Design review of the part built by this model. Coordinates are the model's own, in mm. Give positions to 0.01 mm unless a question says otherwise; leave off trailing zeros. Order: outer loops, then holes, each group sorted by start corner. A loop starts at its lowest first (then second) coordinate and runs counter-clockwise, first axis right, second up. Notation, with made-up numbers: (52, -3) -> (103, -3) arc R32 cw to (103, 28) -> close; hole circle Ø11 at (-31, 53.5). An arc over 180 degrees is marked (long way). Return JSON: item names as keys, results as strings.
```python
from build123d import *

# Parameters (mm, degrees)
SKETCH_1_W          = 31
SKETCH_1_H          = 6
EXTRUDE_1_DEPTH     = 2.5
SKETCH_2_R          = 1.1
CUT_EXTRUDE_1_DEPTH = 32.608171111
SKETCH_3_R          = 0.6
CUT_EXTRUDE_2_DEPTH = 32.608171111
FILLET_1_R          = 2


with BuildPart() as part:
    # 草图1 → 凸台-拉伸1 (new body)
    with BuildSketch(Plane(origin=(0, 0, 0), x_dir=(1, 0, 0), z_dir=(0, 1, 0))):
        with Locations((15.5, -2.64149634)):
            Rectangle(SKETCH_1_W, SKETCH_1_H)
    extrude(amount=EXTRUDE_1_DEPTH)

    # 草图2 → 切除-拉伸1 (cut, through all)
    with BuildSketch(Plane(origin=(0, 2.5, 0), x_dir=(1, 0, 0), z_dir=(0, 1, 0))):
        with Locations(Location((3, -2.64149634, 0), (0, 0, 270))):
            Circle(SKETCH_2_R)
        with Locations(Location((17, -2.64149634, 0), (0, 0, 270))):
            Circle(SKETCH_2_R)
    extrude(amount=-CUT_EXTRUDE_1_DEPTH, mode=Mode.SUBTRACT)

    # 草图3 → 切除-拉伸2 (cut, through all)
    with BuildSketch(Plane(origin=(0, 2.5, 0), x_dir=(1, 0, 0), z_dir=(0, 1, 0))):
        with Locations(Location((28.5, -2.64149634, 0), (0, 0, 270))):
            Circle(SKETCH_3_R)
    extrude(amount=-CUT_EXTRUDE_2_DEPTH, mode=Mode.SUBTRACT)

    # 圆角1
    fillet_1_edges = [part.edges().sort_by_distance(p)[0] for p in [
        (0, 1.25, -0.35850366),
        (31, 1.25, -0.35850366),
        (31, 1.25, 5.64149634),
        (0, 1.25, 5.64149634),
    ]]
    fillet(fillet_1_edges, radius=FILLET_1_R)


solid = part.part
```
Item 1: For pin 1 (1 mm diameter, centred on x = 28.5, z = 2.64, fed in from +Y), flat-tipped, find the tip position at first contact; note if it passes through.
Result set:
{"pin 1": "passes through"}
Item 2: Add section C-C (y = 0.35). Give the boundary of the cut face in (x, z).
Result set:
{"outline": "(0, 1.64) arc R2 ccw to (2, -0.36) -> (29, -0.36) arc R2 ccw to (31, 1.64) -> (31, 3.64) arc R2 ccw to (29, 5.64) -> (2, 5.64) arc R2 ccw to (0, 3.64) -> close; hole circle Ø2.2 at (3, 2.64); hole circle Ø2.2 at (17, 2.64); hole circle Ø1.2 at (28.5, 2.64)"}
Item 3: Mouldability with a two-part tool opening along X and no side actions: class faces 1 (the face through (15, 1, 5.641)), 2 (the face through (0.57, 1.27, 5.04)), 3 (the face through (3.74, 1.27, 1.83)) as released by +X, released by -X, zero draft, split by the parting line, or undercut.
Result set:
{"face 1": "zero draft", "face 2": "released by -X", "face 3": "undercut"}
Item 4: Wall thickness on L1, parallel to X at y = 1.6, z = 2.75; L2, parallel to X at y = 1.4, z = 2.4; L3, parallel to X at y = 0.3, z = 3.4: over which ranges is each line inside the solid? List them lowest first. Write a range as [from, to].
Result set:
{"L1": "x = [0, 1.91], [4.09, 15.91], [18.09, 27.91], [29.09, 31]", "L2": "x = [0, 1.93], [4.07, 15.93], [18.07, 27.95], [29.05, 31]", "L3": "x = [0, 2.2], [3.8, 16.2], [17.8, 31]"}
Item 5: Add section D-D (x = 3). Give the boundary of the cut face in (y, z), plus the area to 3 significant figures.
Result set:
{"outline": "(0, -0.36) -> (2.5, -0.36) -> (2.5, 1.54) -> (0, 1.54) -> close; (0, 3.74) -> (2.5, 3.74) -> (2.5, 5.64) -> (0, 5.64) -> close", "area": "9.50 mm^2"}
Item 6: Add section A-A (x = 28.5). Give the boundary of the cut face in (y, z).
Result set:
{"outline": "(0, -0.36) -> (2.5, -0.36) -> (2.5, 2.04) -> (0, 2.04) -> close; (0, 3.24) -> (2.5, 3.24) -> (2.5, 5.64) -> (0, 5.64) -> close"}
Item 7: Add section B-B (z = 2.7). Give the boundary of the cut face in (x, y).
Result set:
{"outline": "(0, 0) -> (1.9, 0) -> (1.9, 2.5) -> (0, 2.5) -> close; (4.1, 0) -> (15.9, 0) -> (15.9, 2.5) -> (4.1, 2.5) -> close; (18.1, 0) -> (27.9, 0) -> (27.9, 2.5) -> (18.1, 2.5) -> close; (29.1, 0) -> (31, 0) -> (31, 2.5) -> (29.1, 2.5) -> close"}
